Input: dimensioned drawing with shaded views. Units: mm. Origin: part minimum x, y, z. A direction names the side the tool comes from. Give positions to 0.01 mm unless a question says otherwise; leave off trailing zeros. Write each loop counter-clockwise with the first axis right and the second up, starting at its lowest first coordinate (ties: lowest second). Pieces come first, ordered by that corner, then holes. Notation, with made-up numbers: M 12,-16 L 20,-16 A16 cw 20,-9 Z; hole C -26.75,45.25 d3. An arc over 180 degrees is marked long. Answer as a JSON object with one key per item and string values.
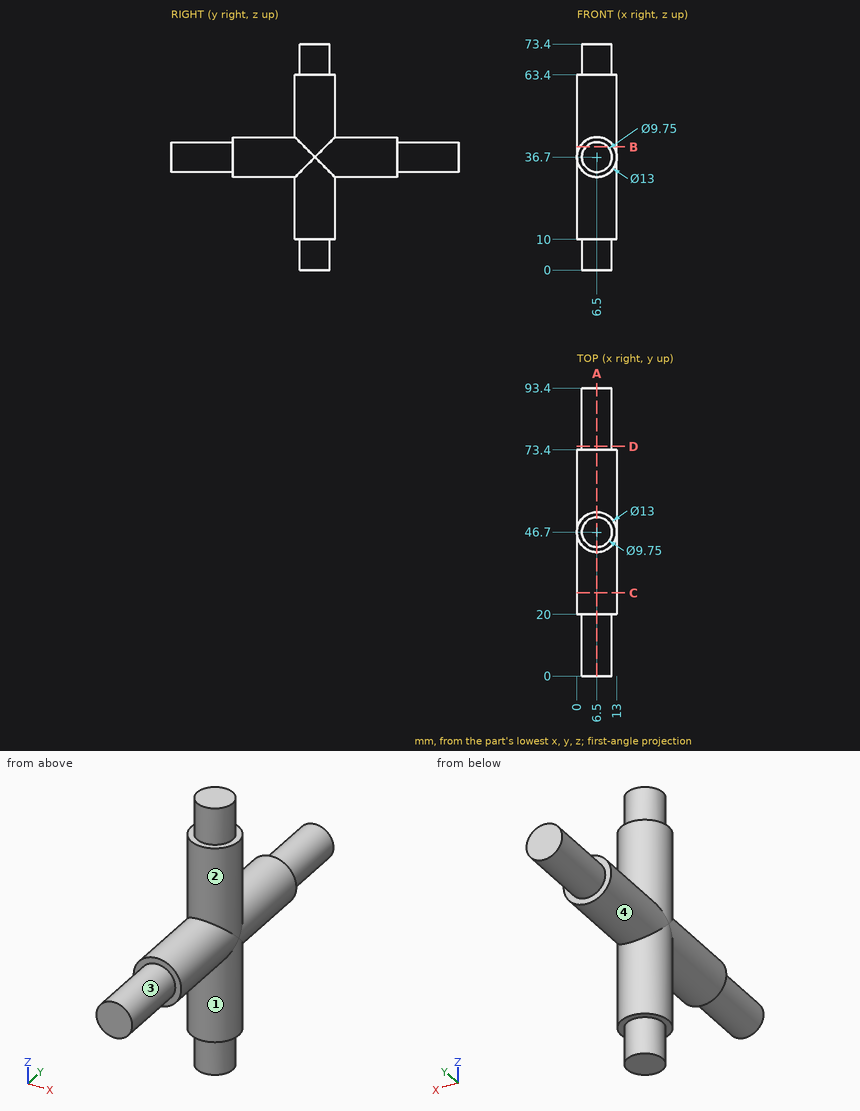
1) Contact query for a flat-ended pin moving along its axis: P1, Ø6, axis at y = 56.5, z = 42, coming from the -X side. Output: stop coordinate, or through.
Geometry check:
{"P1": "stops at x = 0.42"}
2) Set-up query: the marked faces 1, 2, 3 and 4. Return all of +Z, -Z, +X, -X, +Y, -Y with unobstructed straight access to the full face (end or side cutting, diameter ignored); none if empty.
Geometry check:
{"face 1": "-Z", "face 2": "+Z", "face 3": "-Y", "face 4": "+Y"}
3) Line query: line 1 (Y direction, x = 12, z = 38); line 2 (Z direction, x = 4.75, y = 35); line 3 (Z direction, x = 5, y = 42). Output: solid intervals per line, ascending. Write a range as from..to.
Geometry check:
{"line 1": "y = 20..73.4", "line 2": "z = 30.44..42.96", "line 3": "z = 10..63.4"}
4) Cut plane B-B on z = 40. Return loops of the section in (x, y), and give its area (3 significant figures).
Geometry check:
{"outline": "M 0.9,20 L 2.91,20 L 2.91,0 L 10.09,0 L 10.09,20 L 12.1,20 L 12.1,43.4 A6.5 ccw 12.1,50 L 12.1,73.4 L 10.09,73.4 L 10.09,93.4 L 2.91,93.4 L 2.91,73.4 L 0.9,73.4 L 0.9,50 A6.5 ccw 0.9,43.4 Z", "area": "893 mm2"}
5) Cut plane A-A on x = 6.5. Return loops of the section in (y, z) (3 decimals).
Geometry check:
{"outline": "M 0,31.825 L 20,31.825 L 20,30.2 L 40.2,30.2 L 40.2,10 L 41.825,10 L 41.825,0 L 51.575,0 L 51.575,10 L 53.2,10 L 53.2,30.2 L 73.4,30.2 L 73.4,31.825 L 93.4,31.825 L 93.4,41.575 L 73.4,41.575 L 73.4,43.2 L 53.2,43.2 L 53.2,63.4 L 51.575,63.4 L 51.575,73.4 L 41.825,73.4 L 41.825,63.4 L 40.2,63.4 L 40.2,43.2 L 20,43.2 L 20,41.575 L 0,41.575 Z"}
6) Cut plane D-D on y = 74.5. Return loops of the section in (x, z) (3 decimals).
Geometry check:
{"outline": "C 6.5,36.7 d9.75"}
7) Cut plane C-C on y = 27. Return loops of the section in (x, z).
Geometry check:
{"outline": "C 6.5,36.7 d13"}
